Source: CAD feature listing. Evaluate the final solid. Frame: model axes, mm. A direction names the side the tool comes from. Coordinates: 2 decimals unless noted, no trailing zeros. Write each loop counter-clockwise with the first axis right and the second up, starting at its lowest first coordinate (ties: lowest second). Pieces come first, ordered by that corner, then holes. Notation, with made-up numbers: M -17.75,-30.75 L 15.25,-30.75 A16 cw 15.25,-3.75 Z; hole C 23,24.5 d4. An arc over 180 degrees is marked long. Write item = value, one per line. Start each with the question number.
1. Section query A-A (z = 0). Output: boundary loops of the cut face in (x, y), then the cut area to 3 significant figures.
2. Pull-direction query (X, two-part tool) for faces 4 (the face through (-6.676, 92.688, -0.105)), 5 (the face through (-0.391, 44.474, -6.74)), 6 (the face through (0, 21, -7.5)); classes: pulls with the +X half, pulls with the -X half, needs draft (parallel to the pull), parting line crosses it, or undercut.
3. Section query C-C (x = -0.25). Output: boundary loops of the cut face in (y, z), then the cut area to 3 significant figures.
4. Access query for faces 1 (the face through (-6, 20, 0)), 2 (the face through (0, -50, 7)), 3 (the face through (6.54, 86.24, -0.11)). Directions: +Z, -Z, +X, -X, +Y, -Y. A direction counts if a zero-diameter tool reaches every point of the face in a straight line with its end or side. Return the directions, or none.
5. Line query: line 1 along Z through (x, y) = (3.5, -2); line 2 along Y through (x, z) = (0, 6.7). Output: solid intervals per line, ascending.
6. Section query B-B (y = 41.5). Output: boundary loops of the cut face in (x, z).
7. Pin query (flat end, axial travel): pin 1 Ø3 at (x, z) = (-1.5, 5.5) entering from +Y; pin 2 Ø1.5 at (x, z) = (5.5, -2.5) entering from +Y; pin 3 Ø3.5 at (x, y) = (0, 41.5) entering from -Z; pin 4 Ø8 at (x, z) = (1.5, -4.5) entering from +Y. Return the tip coordinate at first contact, or that it passes through.
Solid Edge part; units mm, degrees
sketch "Sketch1" plane through (0, 0, 0) normal (0, -1, 0) x (1, 0, 0)
  line L0 (-6, 6) -> (-6, -6)
  line L1 (-6, -6) -> (6, -6)
  line L2 (6, -6) -> (6, 6)
  line L3 (6, 6) -> (-6, 6)
  line L4 (-7.5, 7.5) -> (-7.5, -7.5)
  line L5 (-7.5, -7.5) -> (7.5, -7.5)
  line L6 (7.5, -7.5) -> (7.5, 7.5)
  line L7 (7.5, 7.5) -> (-7.5, 7.5)
extrude "ExtrudedProtrusion_1" add sketch "Sketch1" against normal blind 94 and the other way blind 50
sketch "Sketch2" plane through (0, 0, 0) normal (0, 0, 1) x (1, 0, 0)
  circle A0 centre (0, 41.5) radius 3
  circle A1 centre (0, -41.5) radius 3
extrude "Cutout1" cut sketch "Sketch2" along normal up to next and the other way up to next
sketch "Sketch3" plane through (0, 0, 0) normal (0, 0, 1) x (1, 0, 0)
  line L0 (-46.6431, 82.7984) -> (-4.4565, 93.2369)
  line L1 (-4.4565, 93.2369) -> (4.1313, 85.3647)
  line L2 (4.1313, 85.3647) -> (32.2719, 95.6112)
extrude "Cutout2" cut sketch "Sketch3" along normal up to next and the other way up to next material side at (-25.5618, 88.0662, 0)
Results are:
q1.outline = M -7.5,-50 L -6,-50 L -6,92.85 L -7.5,92.48 Z; M 6,-50 L 7.5,-50 L 7.5,86.59 L 6,86.05 Z
q1.area = 418 mm^2
q2.face_4 = pulls with the -X half
q2.face_5 = undercut
q2.face_6 = needs draft
q3.outline = M -50,-7.5 L -44.49,-7.5 L -44.49,-6 L -50,-6 Z; M -50,6 L -44.49,6 L -44.49,7.5 L -50,7.5 Z; M -38.51,-7.5 L 38.51,-7.5 L 38.51,-6 L -38.51,-6 Z; M -38.51,6 L 38.51,6 L 38.51,7.5 L -38.51,7.5 Z; M 44.49,-7.5 L 89.38,-7.5 L 89.38,-6 L 44.49,-6 Z; M 44.49,6 L 89.38,6 L 89.38,7.5 L 44.49,7.5 Z
q3.area = 382 mm^2
q4.face_1 = +Y, -Y
q4.face_2 = +Z, -Z, +X, -X, -Y
q4.face_3 = +Z, -Z, +Y
q5.line_1 = -7.5 to -6, 6 to 7.5
q5.line_2 = -50 to -44.5, -38.5 to 38.5, 44.5 to 89.15
q6.outline = M -7.5,-7.5 L -3,-7.5 L -3,-6 L -6,-6 L -6,6 L -3,6 L -3,7.5 L -7.5,7.5 Z; M 3,-7.5 L 7.5,-7.5 L 7.5,7.5 L 3,7.5 L 3,6 L 6,6 L 6,-6 L 3,-6 Z
q7.pin_1 = 91.82
q7.pin_2 = 86.14
q7.pin_3 = through
q7.pin_4 = 91.18
